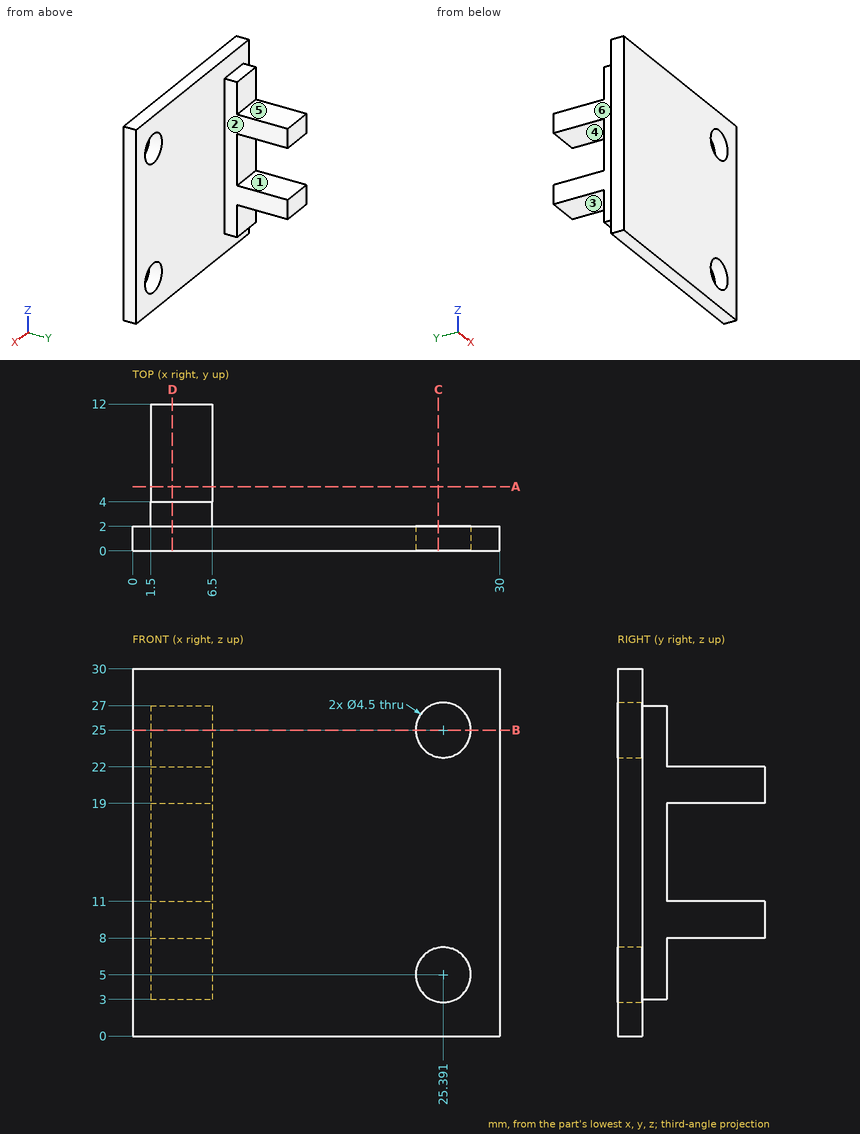
Part print with two shaded views. Sizes in mm from the minimum x, y, z corner. A direction names the side the tool comes from. Round coordinates to 2 decimals unless told otherwise and drop trailing zeros. Order: outer loops, then holes, each group sorted by start corner. A loop starts at its lowest first (then second) coordinate and runs counter-clockwise, first axis right, second up. Notation, with made-up numbers: (-6.5, 81.25) - (50.5, 81.25) arc R24 cw to (50.5, 119.25) - close; hole circle Ø5 at (-27, 67.25). An arc over 180 degrees is marked (long way). Answer as CSV lines item,"result". Start each with the question number.
1. Pin check, flat tips, straight feed: pin 1 (5.5 mm diameter, centred on x = 4, y = 8.5, fed in from +Z); pin 2 (4 mm diameter, centred on x = 9.5, z = 14, fed in from +Y); pin 3 (4 mm diameter, centred on x = 4.5, z = 16, fed in from +Y); pin 4 (6 mm diameter, centred on x = 17.5, y = 5.5, fed in from +Z). Stop position of each tip, or through.
2. Pull direction Z, two halves, no side cores. Call the marked faces 4, 5 and 6: +Z half, -Z half, draft (parallel to the pull), parting line (faces both ways), or undercut.
3. Drill centre lines: L1, parallel to X at y = 0.85, z = 5; L2, parallel to Z at x = 3.75, y = 8.75; L3, parallel to Y at x = 11.5, z = 19.25. Where is each one in solid material? Low to high. Write a range as [from, to].
4. Tool access for the marked faces 1, 2 and 3: list every direction of +Z, -Z, +X, -X, +Y, -Y with a clear straight run to the whole face (end or side of a thin tool).
5. Saw through at C-C, the plane x = 25. Write the cut outline in (y, z).
6. Saw through at D-D, the plane x = 3.25. Write the cut outline in (y, z).
7. Saw through at A-A, the plane y = 5.25. Write the cut outline in (x, z), and give its area (3 significant figures).
8. Saw through at B-B, the plane z = 25. Write the cut outline in (x, y), and give its area (3 significant figures).
Model answer:
1,pin 1,"stops at z = 22"
1,pin 2,"stops at y = 2"
1,pin 3,"stops at y = 4"
1,pin 4,"passes through"
2,face 4,"undercut"
2,face 5,"+Z half"
2,face 6,"draft"
3,L1,"x = [0, 23.14], [27.64, 30]"
3,L2,"z = [8, 11], [19, 22]"
3,L3,"y = [0, 2]"
4,face 1,"+X, -X, +Y"
4,face 2,"+Z, -Z, +X, +Y"
4,face 3,"-Z, +X, -X, +Y"
5,outline,"(0, 0) - (2, 0) - (2, 2.78) - (0, 2.78) - close; (0, 7.22) - (2, 7.22) - (2, 22.78) - (0, 22.78) - close; (0, 27.22) - (2, 27.22) - (2, 30) - (0, 30) - close"
6,outline,"(0, 0) - (2, 0) - (2, 3) - (4, 3) - (4, 8) - (12, 8) - (12, 11) - (4, 11) - (4, 19) - (12, 19) - (12, 22) - (4, 22) - (4, 27) - (2, 27) - (2, 30) - (0, 30) - close"
7,outline,"(1.5, 8) - (6.5, 8) - (6.5, 11) - (1.5, 11) - close; (1.5, 19) - (6.5, 19) - (6.5, 22) - (1.5, 22) - close"
7,area,"30.0 mm²"
8,outline,"(0, 0) - (23.14, 0) - (23.14, 2) - (6.5, 2) - (6.5, 4) - (1.5, 4) - (1.5, 2) - (0, 2) - close; (27.64, 0) - (30, 0) - (30, 2) - (27.64, 2) - close"
8,area,"61.0 mm²"
